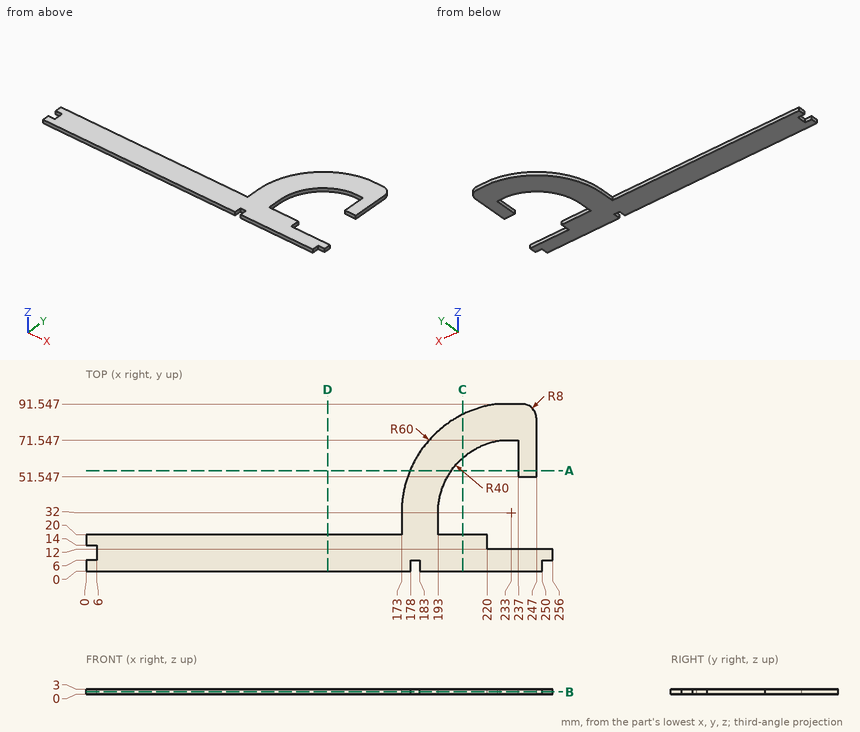
Geometry: see drawing. Coordinates: mm, zero at the bounding-box minimum. Give positions to 0.01 mm unless a question says otherwise; leave off trailing zeros. Write each loop counter-clockwise with the first axis right and the second up, starting at its lowest first coordinate (ties: lowest second). Pieces come first, ordered by that corner, then holes. Notation, with made-up numbers: (-7.75, 87) -> (-0.75, 87) arc R5 ccw to (-0.75, 93) -> close; hole circle Ø3 at (44, 45.5). An arc over 180 degrees is marked (long way). Use one line per item in the form item = value. Start each with the question number.
1) Section query C-C on x = 206.5. Return the cut outline in (y, z), then the cut area to 3 significant figures.
2) Pin query (flat end, axial travel): pin 1 (0.9 mm diameter, centred on x = 3, z = 1, fed in from -Y); pin 2 (0.9 mm diameter, centred on x = 253.5, z = 1, fed in from -Y); pin 3 (1.5 mm diameter, centred on y = 37.5, z = 1.5, fed in from -X); pin 4 (1.5 mm diameter, centred on y = 63, z = 1, fed in from +X). Return the tip coordinate at first contact, or that it passes through.
3) Ray query, probe 1 along Y at (x, z) = (114, 2.7); probe 2 along X at (y, z) = (56, 0.35); probe 3 along X at (y, z) = (34, 2.25). Return the intervals inside material, ascending. Write a range as from..to.
4) Section query A-A on y = 55. Return the cut outline in (x, z).
5) Section query B-B on z = 1.4. Return the cut outline in (x, y) (1 decimal).
6) Section query D-D on x = 132.5. Return the cut outline in (y, z), then the cut area to 3 significant figures.
Outcome:
q1.outline = (0, 0) -> (20, 0) -> (20, 3) -> (0, 3) -> close; (61.96, 0) -> (85.83, 0) -> (85.83, 3) -> (61.96, 3) -> close
q1.area = 132 mm^2
q2.pin_1 = 0
q2.pin_2 = 6
q2.pin_3 = 173.19
q2.pin_4 = 247
q3.probe_1 = 0..20
q3.probe_2 = 178.01..201, 237..247
q3.probe_3 = 173.03..193.05
q4.outline = (177.58, 0) -> (200.27, 0) -> (200.27, 3) -> (177.58, 3) -> close; (237, 0) -> (247, 0) -> (247, 3) -> (237, 3) -> close
q5.outline = (0, 0) -> (178, 0) -> (178, 6) -> (183, 6) -> (183, 0) -> (250, 0) -> (250, 6) -> (256, 6) -> (256, 12) -> (220, 12) -> (220, 20) -> (193, 20) -> (193, 32) arc R40 cw to (227, 71.5) -> (237, 71.5) -> (237, 51.5) -> (247, 51.5) -> (247, 83.5) arc R8 ccw to (239, 91.5) -> (225.6, 91.5) arc R60 ccw to (173, 32) -> (173, 20) -> (0, 20) -> (0, 14) -> (6, 14) -> (6, 6) -> (0, 6) -> close
q6.outline = (0, 0) -> (20, 0) -> (20, 3) -> (0, 3) -> close
q6.area = 60.0 mm^2
